CAD build for the part. Positions are in the model's coordinates, mm. A direction names the side the tool comes from. Round coordinates to 2 decimals unless told otherwise and drop trailing zeros. Order: outer loops, then holes, each group sorted by start corner. A loop starts at its lowest first (then second) coordinate and runs counter-clockwise, first axis right, second up. Notation, with made-up numbers: M 73.25,-7.75 L 117.25,-7.75 A18 cw 117.25,10.25 Z; hole C 86,74.25 d10. An arc over 180 degrees is marked long. Answer as a JSON object with one key per item and string values.
```python
from build123d import *

# Parameters (mm, degrees)
BOSS_EXTRUDE1_DEPTH      = 27
BOSS_EXTRUDE1_DEPTH_BACK = 27
CUT_EXTRUDE1_START       = -8
SKETCH4_W                = 46
SKETCH4_H                = 54
CUT_EXTRUDE1_DEPTH       = 76.779472426
SKETCH5_R                = 3
CUT_EXTRUDE2_DEPTH       = 84.779472426
SKETCH6_R                = 2
CUT_EXTRUDE4_DEPTH       = 10


with BuildPart() as part:
    # Sketch1 → Boss-Extrude1 (new, two sides: drawn at the far end of the back side and taken through both)
    with BuildSketch(Plane(origin=(0, 0, 0), x_dir=(0, 0, -1), z_dir=(1, 0, 0)).offset(-BOSS_EXTRUDE1_DEPTH_BACK)):
        Polygon((0, 31), (0, -31), (73, -31), (73, -23), (8, 31), align=None)
    extrude(amount=BOSS_EXTRUDE1_DEPTH + BOSS_EXTRUDE1_DEPTH_BACK)

    # Sketch4 → Cut-Extrude1 (cut, through all)
    with BuildSketch(Plane.XY.offset(CUT_EXTRUDE1_START)):
        with Locations((0, 4)):
            Rectangle(SKETCH4_W, SKETCH4_H)
    extrude(amount=-CUT_EXTRUDE1_DEPTH, mode=Mode.SUBTRACT)

    # Sketch5 → Cut-Extrude2 (cut, through all)
    with BuildSketch(Plane(origin=(0, 0, 0), x_dir=(-1, 0, 0), z_dir=(0, 0, -1))):
        with Locations(Location((17.67766953, 17.67766953, 0), (0, 0, 180))):
            Circle(SKETCH5_R)
        with Locations(Location((17.67766953, -17.67766953, 0), (0, 0, 180))):
            Circle(SKETCH5_R)
        with Locations(Location((-17.67766953, -17.67766953, 0), (0, 0, 180))):
            Circle(SKETCH5_R)
        with Locations(Location((-17.67766953, 17.67766953, 0), (0, 0, 180))):
            Circle(SKETCH5_R)
    extrude(amount=CUT_EXTRUDE2_DEPTH, mode=Mode.SUBTRACT)

    # Sketch6 → Cut-Extrude4 (cut)
    with BuildSketch(Plane(origin=(0, -31, -35), x_dir=(1, 0, 0), z_dir=(0, 1, 0))):
        with Locations(Location((0, -21, 0), (0, 0, 90))):
            Circle(SKETCH6_R)
        with Locations(Location((0, 24, 0), (0, 0, 90))):
            Circle(SKETCH6_R)
        with Locations(Location((18, 1.5, 0), (0, 0, 90))):
            Circle(SKETCH6_R)
        with Locations(Location((-18, 1.5, 0), (0, 0, 90))):
            Circle(SKETCH6_R)
    extrude(amount=CUT_EXTRUDE4_DEPTH, mode=Mode.SUBTRACT)


solid = part.part
```
Item 1: Drop flat-ended pins along their axis: pin 1 Ø3.5 at (x, y) = (-17.68, 17.68) entering from -Z; pin 2 Ø9.5 at (x, y) = (17.68, 17.68) entering from -Z; pin 3 Ø12 at (x, z) = (1.5, -36) entering from +Y. Give the stop position or say it passes through.
Worked answers:
{"pin 1": "passes through", "pin 2": "stops at z = -8", "pin 3": "stops at y = -23"}
Item 2: Wall check: line 1 along X through (y, z) = (-29, -59); line 2 along X through (y, z) = (-27, -36.5); line 3 along Z through (x, y) = (18, -28). Give the ranges that are in metal, low to high. Write a range as [from, to].
Worked answers:
{"line 1": "x = [-27, -2], [2, 27]", "line 2": "x = [-27, -20], [-16, 16], [20, 27]", "line 3": "z = [-73, -38.5], [-34.5, 0]"}
Item 3: Saw through at B-B on z = -36.5. List the corners of the cut face in (x, y), and give its area (3 significant figures).
Worked answers:
{"outline": "M -27,-31 L -20,-31 L -20,-23 L -23,-23 L -23,7.32 L -27,7.32 Z; M -16,-31 L 16,-31 L 16,-23 L -16,-23 Z; M 20,-31 L 27,-31 L 27,7.32 L 23,7.32 L 23,-23 L 20,-23 Z", "area": "611 mm2"}
Item 4: Saw through at D-D on x = 18. List the corners of the cut face in (y, z).
Worked answers:
{"outline": "M -31,-73 L -23,-73 L -23,-38.5 L -31,-38.5 Z; M -31,-34.5 L -23,-34.5 L -23,-8 L -20.66,-8 L -20.66,0 L -31,0 Z; M -14.7,-8 L 14.7,-8 L 14.7,0 L -14.7,0 Z; M 20.66,-8 L 31,-8 L 31,0 L 20.66,0 Z"}
Item 5: 3-axis set-ups, long thin cutter, end or side, ignore diameter. For faces 1 (the cylindrical face through (-20.058, -15.852, -3.944)), 2 (the flat face through (0, 4, -8)): which of +Z, -Z, +X, -X, +Y, -Y reach the whole face in a straight line?
Worked answers:
{"face 1": "+Z, -Z", "face 2": "-Z, +Y"}
Item 6: Saw through at C-C on z = -14. List the corners of the cut face in (x, y).
Worked answers:
{"outline": "M -27,-31 L -2,-31 L -2,-23 L -23,-23 L -23,26.02 L -27,26.02 Z; M 2,-31 L 27,-31 L 27,26.02 L 23,26.02 L 23,-23 L 2,-23 Z"}
Item 7: Saw through at A-A on x = 0. List the corners of the cut face in (y, z).
Worked answers:
{"outline": "M -31,-73 L -23,-73 L -23,-61 L -31,-61 Z; M -31,-57 L -23,-57 L -23,-16 L -31,-16 Z; M -31,-12 L -23,-12 L -23,-8 L 31,-8 L 31,0 L -31,0 Z"}
Item 8: Two-plate mould, pull along Y, no slides. Class faces 3 (the flat face through (0, -27, -73)), 4 (the cylindrical face through (-20.06, 19.5, -3.94)), 5 (the flat face through (24.972, 3.622, -40.955)), 6 (the cylindrical face through (17, 20.6, -3.9)): released by +Y, released by -Y, zero draft, split by the parting line, or undercut.
Worked answers:
{"face 3": "zero draft", "face 4": "undercut", "face 5": "released by +Y", "face 6": "undercut"}
